Geometry check sheet. Reference: drawing and pictorial views, mm from the part's lowest x, y, z. Round coordinates to 2 decimals unless told otherwise and drop trailing zeros. Loops run counter-clockwise (first coordinate to the right, second up) from the corner with the lowest first, then second, coordinate; pieces in that order, holes last. Notation, with made-up numbers: (9, 37) - (61, 37) arc R26 ccw to (61, 71) - close; hole circle Ø6 at (-9, 61.25). An arc over 180 degrees is marked (long way). Answer as CSV lines item,"result". Start each with the question number.
1) Cross-section at C-C on y = 5. Record the boundary of the cut face in (x, z), and give its area (3 significant figures).
2) Cross-section at A-A on z = 20.05. Record the boundary of the cut face in (x, y).
3) Cross-section at B-B on x = 9.05. Record the boundary of the cut face in (y, z).
4) Thickness scan on line 1 along X through (y, z) = (4.5, 6.05); line 2 along X through (y, z) = (2, 20.05); line 3 along Z through (x, y) = (21.5, 5). Record the ranges inside material, lowest first.
5) Draft check along Z on the marked faces 1, 2, 3 and 4. Enter one of: released by +Z, released by -Z, zero draft, split by the parting line, or undercut.
6) Cross-section at D-D on z = 34.05. Record the boundary of the cut face in (x, y).
7) Depth check by flat-ended pin: P1, Ø6, axis at x = 23, z = 13, coming from the -Y side; P2, Ø16.5, axis at x = 20.2, z = 20.05, coming from the +Y side. Enter the tip coordinate at first touch or a pass-through.
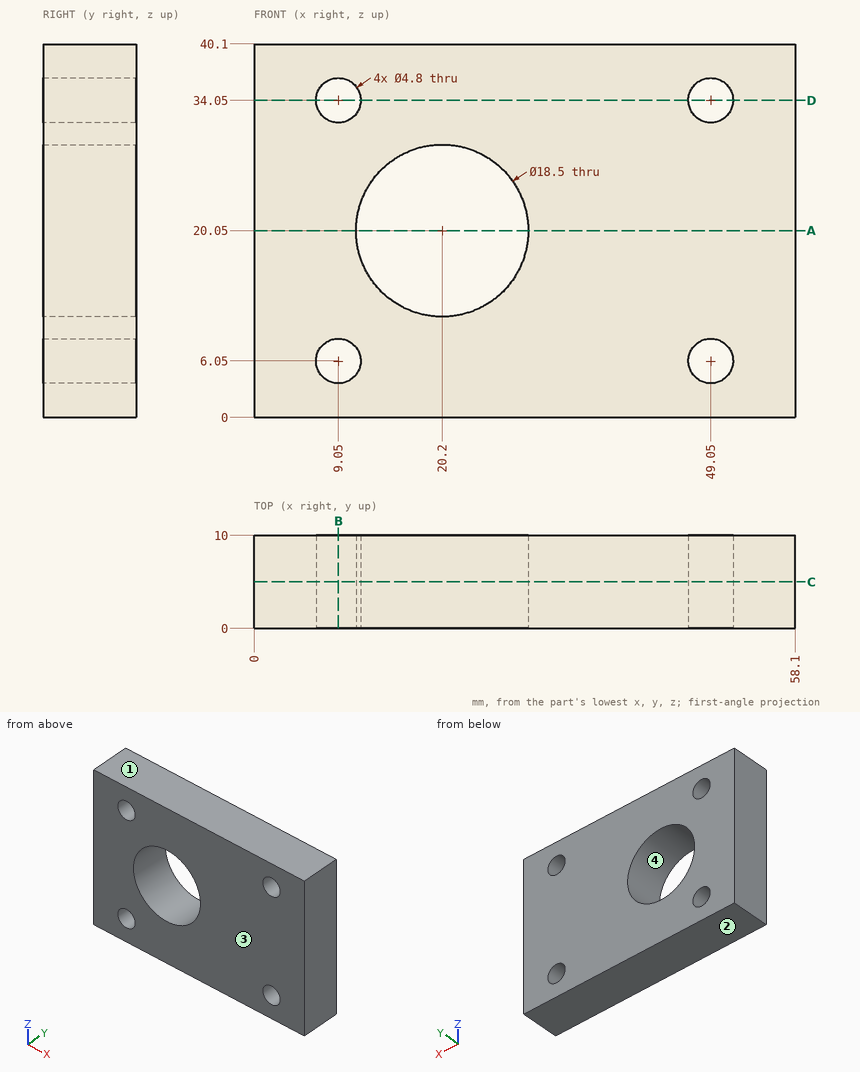
Answer block:
1,outline,"(0, 0) - (58.1, 0) - (58.1, 40.1) - (0, 40.1) - close; hole circle Ø4.8 at (9.05, 6.05); hole circle Ø4.8 at (9.05, 34.05); hole circle Ø18.5 at (20.2, 20.05); hole circle Ø4.8 at (49.05, 6.05); hole circle Ø4.8 at (49.05, 34.05)"
1,area,"1,990 mm^2"
2,outline,"(0, 0) - (10.95, 0) - (10.95, 10) - (0, 10) - close; (29.45, 0) - (58.1, 0) - (58.1, 10) - (29.45, 10) - close"
3,outline,"(0, 0) - (10, 0) - (10, 3.65) - (0, 3.65) - close; (0, 8.45) - (10, 8.45) - (10, 31.65) - (0, 31.65) - close; (0, 36.45) - (10, 36.45) - (10, 40.1) - (0, 40.1) - close"
4,line 1,"x = 0 to 6.65, 11.45 to 46.65, 51.45 to 58.1"
4,line 2,"x = 0 to 10.95, 29.45 to 58.1"
4,line 3,"z = 0 to 10.89, 29.21 to 40.1"
5,face 1,"released by +Z"
5,face 2,"released by -Z"
5,face 3,"zero draft"
5,face 4,"undercut"
6,outline,"(0, 0) - (6.65, 0) - (6.65, 10) - (0, 10) - close; (11.45, 0) - (46.65, 0) - (46.65, 10) - (11.45, 10) - close; (51.45, 0) - (58.1, 0) - (58.1, 10) - (51.45, 10) - close"
7,P1,"stops at y = 0"
7,P2,"passes through"
